Model file for the job. Use its own axes, mm. Face numbers are marked on the shaded views. A direction names the side the tool comes from. Coordinates: 2 decimals unless noted, no trailing zeros. Write each loop counter-clockwise with the first axis right and the second up, starting at its lowest first coordinate (ties: lowest second). Pieces come first, ordered by that corner, then holes. Notation, with made-up numbers: (-5, 9) - (25, 9) arc R22 cw to (25, 44) - close; hole circle Ø8 at (68.5, 1.25). An arc over 180 degrees is marked (long way). Put each result on its own line as item: value. Start each with the question number.
1. Saw through at C-C, the plane x = 15. Write the cut outline in (y, z).
2. Drop flat-ended pins along their axis: P1, Ø3, axis at x = 16, z = -10, coming from the +Y side; P2, Ø5.5, axis at x = 24, z = -10.5, coming from the +Y side; P3, Ø4.5, axis at y = 7.5, z = -12.5, coming from the -X side; P4, Ø5, axis at x = 46, z = -8, coming from the +Y side. Give the stop position or say it passes through.
3. Drill centre lines: L1, parallel to X at y = 7.25, z = -10 (3 decimals); L2, parallel to X at y = 2.65, z = -10 (3 decimals); L3, parallel to X at y = 1.3, z = -10 (3 decimals). Where is each one in solid material? Low to high. Write a range as from..to.
4. Pull direction X, two halves, no side cores. Call the marked faces 4, 5 and 6: released by +X, released by -X, zero draft, split by the parting line, or undercut.
5. Saw through at B-B, the plane x = 34.5. Write the cut outline in (y, z) (3 decimals), plus the area to 3 significant figures.
6. Which spindle directions (+Z, -Z, +X, -X, +Y, -Y) get a long thin tool onto all of the face, cutting with end or side? Do the marked faces 1, 2 and 3. Say none if no direction does.
7. Saw through at A-A, the plane y = 2. Give the number of separate pieces and of enclosed holes in the cut face, plus the area to 3 significant figures.
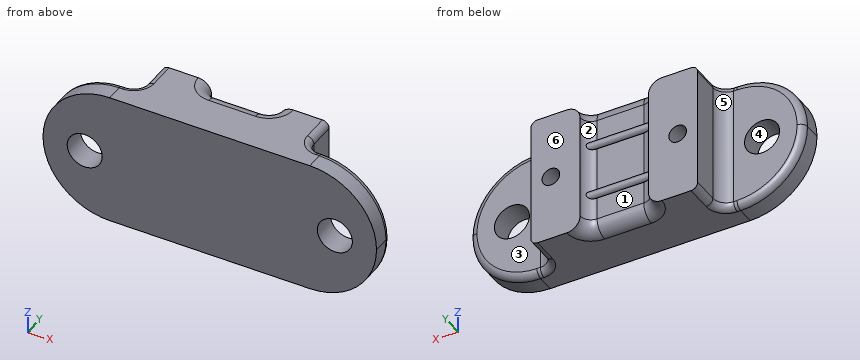
```python
from build123d import *

# Parameters (mm, degrees)
SKETCH1_W           = 50
SKETCH1_H           = 20
BOSS_EXTRUDE1_DEPTH = 3.5
SKETCH2_W           = 25
SKETCH2_H           = 20
BOSS_EXTRUDE2_DEPTH = 6
SKETCH3_R           = 2.625
CUT_EXTRUDE1_DEPTH  = 6
CUT_EXTRUDE2_DEPTH  = 50
SKETCH5_R           = 1.325
CUT_EXTRUDE3_DEPTH  = 7
FILLET1_R           = 10
FILLET2_R           = 2
SKETCH6_R           = 0.625
BOSS_EXTRUDE3_DEPTH = 25
FILLET3_R           = 2
FILLET4_R           = 1


with BuildPart() as part:
    # Sketch1 → Boss-Extrude1 (new body)
    with BuildSketch(Plane(origin=(0, 0, 0), x_dir=(1, 0, 0), z_dir=(0, 1, 0))):
        with Locations((25, 10)):
            Rectangle(SKETCH1_W, SKETCH1_H)
    extrude(amount=BOSS_EXTRUDE1_DEPTH)

    # Sketch2 → Boss-Extrude2 (add)
    with BuildSketch(Plane(origin=(0, 3.5, 0), x_dir=(1, 0, 0), z_dir=(0, 1, 0))):
        with Locations((25, 10)):
            Rectangle(SKETCH2_W, SKETCH2_H)
    extrude(amount=BOSS_EXTRUDE2_DEPTH)

    # Sketch3 → Cut-Extrude1 (cut)
    with BuildSketch(Plane(origin=(0, 3.5, 0), x_dir=(1, 0, 0), z_dir=(0, 1, 0))):
        with Locations(Location((6.25, 10, 0), (0, 0, 270))):
            Circle(SKETCH3_R)
        with Locations(Location((43.75, 10, 0), (0, 0, 270))):
            Circle(SKETCH3_R)
    extrude(amount=-CUT_EXTRUDE1_DEPTH, mode=Mode.SUBTRACT)

    # Sketch4 → Cut-Extrude2 (cut)
    with BuildSketch(Plane.XY):
        with BuildLine():
            Line((21.5, 11.125), (28.5, 11.125))
            ThreePointArc((28.5, 11.125), (30.125, 9.5), (28.5, 7.875))
            Line((28.5, 7.875), (21.5, 7.875))
            ThreePointArc((21.5, 7.875), (19.875, 9.5), (21.5, 11.125))
        make_face()
    extrude(amount=-CUT_EXTRUDE2_DEPTH, mode=Mode.SUBTRACT)

    # Sketch5 → Cut-Extrude3 (cut)
    with BuildSketch(Plane(origin=(0, 9.5, 0), x_dir=(1, 0, 0), z_dir=(0, 1, 0))):
        with Locations(Location((15.5, 10, 0), (0, 0, 270))):
            Circle(SKETCH5_R)
        with Locations(Location((34.5, 10, 0), (0, 0, 270))):
            Circle(SKETCH5_R)
    extrude(amount=-CUT_EXTRUDE3_DEPTH, mode=Mode.SUBTRACT)

    # Fillet1
    fillet1_edges = [part.edges().sort_by_distance(p)[0] for p in [
        (0, 1.75, -20),
        (0, 1.75, 0),
        (50, 1.75, -20),
        (50, 1.75, 0),
    ]]
    fillet(fillet1_edges, radius=FILLET1_R - 0.0001)  # a hair under: the kernel refuses the full size

    # Fillet2
    fillet2_edges = [part.edges().sort_by_distance(p)[0] for p in [
        (12.5, 3.5, -10),
        (37.5, 3.5, -10),
    ]]
    fillet(fillet2_edges, radius=FILLET2_R)

    # Sketch6 → Boss-Extrude3 (add)
    with BuildSketch(Plane(origin=(37.5, 0, 0), x_dir=(0, 0, -1), z_dir=(1, 0, 0))):
        with Locations((6, 7.875)):
            Circle(SKETCH6_R)
        with Locations((14, 7.875)):
            Circle(SKETCH6_R)
    extrude(amount=-BOSS_EXTRUDE3_DEPTH)

    # Fillet3
    fillet3_edges = [part.edges().sort_by_distance(p)[0] for p in [
        (25, 7.875, -20),
        (20.350951481, 8.350951481, -20),
        (29.649048519, 8.350951481, -20),
        (20.350951481, 8.350951481, 0),
        (25, 7.875, 0),
        (29.649048519, 8.350951481, 0),
    ]]
    fillet(fillet3_edges, radius=FILLET3_R)

    # Fillet4
    fillet4_edges = [part.edges().sort_by_distance(p)[0] for p in [
        (12.5, 7.5, -20),
        (12.5, 7.5, 0),
        (37.5, 7.5, 0),
        (37.5, 7.5, -20),
        (39.75005, 3.5, -20),
        (10.24995, 3.5, 0),
        (2.928902899, 3.5, -2.928902899),
        (2.928902899, 3.5, -17.071097101),
        (47.071097101, 3.5, -2.928902899),
        (47.071097101, 3.5, -17.071097101),
        (39.75005, 3.5, 0),
        (10.24995, 3.5, -20),
        (38.085786438, 4.085786438, -20),
        (38.085786438, 4.085786438, 0),
        (11.914213562, 4.085786438, 0),
        (11.914213562, 4.085786438, -20),
    ]]
    fillet(fillet4_edges, radius=FILLET4_R)


solid = part.part
```
Final values:
1. outline: (0, -20) - (9.5, -20) - (9.5, -11.23) - (2.5, -11.23) - (2.5, -8.77) - (9.5, -8.77) - (9.5, 0) - (0, 0) - close
2. P1: stops at y = 9.5
2. P2: stops at y = 7.89
2. P3: stops at x = 12.48
2. P4: stops at y = 3.5
3. L1: x = 12.5..14.175, 16.825..33.175, 35.825..37.5
3. L2: x = 0.011..3.625, 8.875..14.175, 16.825..33.175, 35.825..41.125, 46.375..49.989
3. L3: x = 0..3.625, 8.875..41.125, 46.375..50
4. face 4: undercut
4. face 5: released by -X
4. face 6: zero draft
5. outline: (0, -20) - (9.5, -20) - (9.5, -11.325) - (2.5, -11.325) - (2.5, -8.675) - (9.5, -8.675) - (9.5, 0) - (0, 0) - close
5. area: 171 mm²
6. face 1: -Z, +Y
6. face 2: +Y
6. face 3: +Z, -Z, +X, +Y
7. separate pieces: 1
7. enclosed holes: 2
7. area: 871 mm²
